Read the model definition and answer for the solid it produces. Units are mm, in the model's axes. Face numbers are marked on the shaded views. A direction names the side the tool comes from. Round coordinates to 2 decimals unless told otherwise and drop trailing zeros. Order: outer loops, then holes, each group sorted by start corner. A loop starts at its lowest first (then second) coordinate and runs counter-clockwise, first axis right, second up. Notation, with made-up numbers: (88.25, 45) - (120.25, 45) arc R26 ccw to (120.25, 60) - close; hole circle Ø6 at (-14.5, -7). An arc over 180 degrees is marked (long way). Answer as a JSON object with one key per item and string values. Group by question number.
Q1. A cutting plane is placed at A-A on y = 134. Determine the outline of the cut face in (x, z), and give its area (3 significant figures).
Q2. Consider line 1 (Z direction, x = -25.4, y = 127.75); line 2 (Y direction, x = 10.5, z = -38); line 3 (Y direction, x = -66.5, z = -48). Determine where each line is inside the solid, lowest interval first.
Q3. Given pin 1 Ø9 at (y, z) = (126.5, 6.5) entering from +X; pin 2 Ø6 at (y, z) = (39.5, 23.5) entering from +X; pin 3 Ø5 at (x, z) = (-46.5, -2) entering from +Y, each flat-ended and moving along its own axis, determine where each tip first touches the part or whether it passes through.
Q4. A tool of negligible diameter and unlimited length cuts with its end or side. For the marked faces 1, 2, 3, 4 and 5, from which of +Z, -Z, +X, -X, +Y, -Y can it reach the whole face along a straight path? Write none if from no direction.
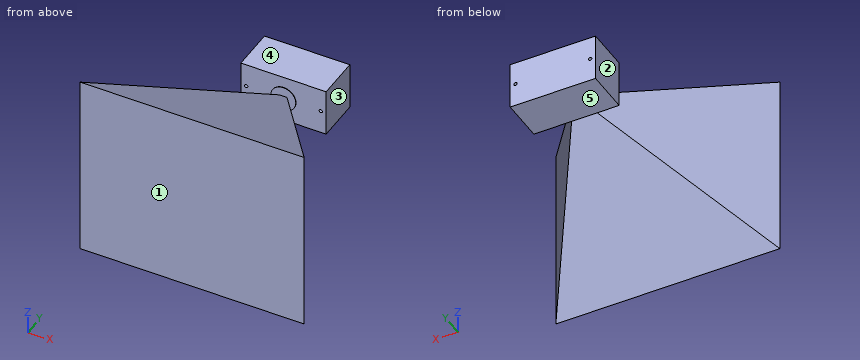
```python
from build123d import *

# Parameters (mm, degrees)
SKETCH3_R                 = 8.509
CAMERA_LENS_DEPTH         = 0.254
SKETCH4_W                 = 58.0644
SKETCH4_H                 = 32.3088
CAMERA_HOLDER_DEPTH       = 29.6672
F_4_40_TAPPED_HOLE1_D     = 2.2606
F_4_40_TAPPED_HOLE1_DEPTH = 29.6672


with BuildPart() as part:
    # Sketch2 → FOV section 0
    with BuildSketch(Plane(origin=(0, 114.3, 0), x_dir=(1, 0, 0), z_dir=(0, 1, 0))):
        with BuildLine():
            Line((-2.473079913, -2.060899928), (2.473079913, -2.060899928))
            Line((2.473079913, -2.060899928), (2.473079913, 2.060899928))
            Line((2.473079913, 2.060899928), (-2.473079913, 2.060899928))
            Line((-2.473079913, 2.060899928), (-2.473079913, -2.060899928))
        make_face()
    # Sketch1 → FOV section 1
    with BuildSketch(Plane(origin=(0, 0, 0), x_dir=(1, 0, 0), z_dir=(0, 1, 0))):
        with BuildLine():
            Line((-76.2, -63.5), (76.2, -63.5))
            Line((76.2, -63.5), (76.2, 63.5))
            Line((76.2, 63.5), (-76.2, 63.5))
            Line((-76.2, 63.5), (-76.2, -63.5))
        make_face()
    loft()

    # Sketch3 → camera lens (add)
    with BuildSketch(Plane(origin=(0, 114.3, 0), x_dir=(1, 0, 0), z_dir=(0, 1, 0))):
        with Locations(Location((0, 0, 0), (0, 0, 270))):
            Circle(SKETCH3_R)
    extrude(amount=CAMERA_LENS_DEPTH)

    # Sketch4 → camera holder (add)
    with BuildSketch(Plane(origin=(0, 114.554, 0), x_dir=(1, 0, 0), z_dir=(0, 1, 0))):
        Rectangle(SKETCH4_W, SKETCH4_H)
    extrude(amount=CAMERA_HOLDER_DEPTH)

    # #4-40 Tapped Hole1
    with Locations(Plane(origin=(0, 144.2212, 0), x_dir=(1, 0, 0), z_dir=(0, 1, 0))):
        with Locations((-25.4, 0), (25.4, 0)):
            Hole(F_4_40_TAPPED_HOLE1_D / 2, depth=F_4_40_TAPPED_HOLE1_DEPTH)


solid = part.part
```
Result set:
{
 "1": {"outline": "(-29.03, -16.15) - (29.03, -16.15) - (29.03, 16.15) - (-29.03, 16.15) - close; hole circle Ø2.26 at (-25.4, 0); hole circle Ø2.26 at (25.4, 0)", "area": "1,870 mm²"},
 "2": {"line 1": "z = -16.15 to -1.13, 1.13 to 16.15", "line 2": "y = 0 to 47.44", "line 3": "y = 0 to 15.04"},
 "3": {"pin 1": "stops at x = 29.03", "pin 2": "stops at x = 52.66", "pin 3": "stops at y = 49.92"},
 "4": {"face 1": "+Z, -Z, +X, -X, -Y", "face 2": "+Z, -Z, -X, +Y", "face 3": "+Z, -Z, +X, +Y", "face 4": "+Z, +X, -X, +Y", "face 5": "-Z, +X, -X, +Y"}
}
